Read the model definition and answer for the solid it produces. Units are mm, in the model's axes. Round coordinates to 2 decimals unless told otherwise and drop trailing zeros. Order: outer loops, then holes, each group sorted by start corner. A loop starts at its lowest first (then second) coordinate and runs counter-clockwise, first axis right, second up. Notation, with made-up numbers: (-6.5, -35.5) -> (-0.5, -35.5) arc R17 ccw to (-0.5, -11.5) -> close; hole circle Ø7 at (-5.75, 61.5). An arc over 180 degrees is marked (long way). Answer as a JSON object with one key per item and string values. Group by question number.
Item 1: Section A-A, the plane y = 0.05 is taken. Write down the section's boundary in (x, z).
Item 2: Consider probe 1 along X at (y, z) = (-0.8, 0.25); probe 2 along Z at (x, y) = (1.5, -0.6); probe 3 along X at (y, z) = (-0.55, 0.75). Determine where each line is inside the solid, lowest interval first. Write a range as from..to.
Item 3: Section C-C, the plane x = 0.25 is taken. Write down the section's boundary in (y, z).
Item 4: Section B-B, the plane z = 2.8 is taken. Write down the section's boundary in (x, y), plus the area to 3 significant figures.
Item 5: Section D-D, the plane x = -3 is taken. Write down the section's boundary in (y, z).
from build123d import *

# Parameters (mm, degrees)
F0_W     = 10
F0_H     = 3
F1_DEPTH = 3
F3_DEPTH = 25
F4_SIZE  = 1


with BuildPart() as f1:
    # F0 (on Top) → F1 (new body)
    with BuildSketch(Plane.XY):
        Rectangle(F0_W, F0_H)
    extrude(amount=F1_DEPTH)

    # F2 (on face) → F3 (cut)
    with BuildSketch(Plane.XZ.offset(1.5)):
        Polygon((-5, 3), (-5, 1), (2, 3), align=None)
    extrude(amount=-F3_DEPTH, mode=Mode.SUBTRACT)

    # F4
    f4_edges = [f1.edges().sort_by_distance(p)[0] for p in [
        (5, 0, 3),
        (5, -1.5, 1.5),
        (5, 1.5, 1.5),
    ]]
    chamfer(f4_edges, length=F4_SIZE)


solid = f1.part
Values found:
{
 "1": {"outline": "(-5, 0) -> (5, 0) -> (5, 2) -> (4, 3) -> (2, 3) -> (-5, 1) -> close"},
 "2": {"probe 1": "-5..4.7", "probe 2": "0..2.86", "probe 3": "-5..4.95"},
 "3": {"outline": "(-1.5, 0) -> (1.5, 0) -> (1.5, 2.5) -> (-1.5, 2.5) -> close"},
 "4": {"outline": "(1.3, -1.5) -> (4, -1.5) -> (4.2, -1.3) -> (4.2, 1.3) -> (4, 1.5) -> (1.3, 1.5) -> close", "area": "8.66 mm2"},
 "5": {"outline": "(-1.5, 0) -> (1.5, 0) -> (1.5, 1.57) -> (-1.5, 1.57) -> close"}
}
